Design review of the part built by this model. Coordinates are the model's own, in mm. Give positions to 0.01 mm unless a question says otherwise; leave off trailing zeros. Order: outer loops, then holes, each group sorted by start corner. A loop starts at its lowest first (then second) coordinate and runs counter-clockwise, first axis right, second up. Notation, with made-up numbers: (7.25, -24.5) -> (14.25, -24.5) arc R10 cw to (14.25, -6.5) -> close; hole circle Ø6 at (49, 41). An arc over 180 degrees is marked (long way). One line per item, written item: value. Start each with the question number.
1) Wall thickness on line 1 along X through (y, z) = (18, 0.45); line 2 along Y through (x, z) = (-154, 0.65); line 3 along X through (y, z) = (10, 1.9): over which ranges is each line inside the solid? List them lowest first. Write a range as from..to.
2) Consider section C-C (z = 2.4). State how many separate pieces and enclosed holes the cut face has, plus the area to 3 significant figures.
3) Consider section B-B (x = -20). State the section outline as (y, z) points.
4) Consider section A-A (y = 17.5). State the section outline as (x, z) points, plus the area to 3 significant figures.
Autodesk Fusion 360 part; units mm, degrees
sketch "plate-2026-03-03T15_18_35.082Z" plane through (0, 0, 0) normal (0, 0, 1) x (1, 0, 0)
  line L0 (-7.0864, -44.9336) -> (-7.0864, -31.9336)
  line L1 (6.9136, -44.9336) -> (6.9136, -31.9336)
  line L2 (-6.5864, -45.4336) -> (6.4136, -45.4336)
  line L3 (-6.5864, -31.4336) -> (6.4136, -31.4336)
  arc A0 (-7.0864, -44.9336) -> (-6.5864, -45.4336) centre (-6.5864, -44.9336) ccw
  arc A1 (-6.5864, -31.4336) -> (-7.0864, -31.9336) centre (-6.5864, -31.9336) ccw
  arc A2 (6.4136, -45.4336) -> (6.9136, -44.9336) centre (6.4136, -44.9336) ccw
  arc A3 (6.9136, -31.9336) -> (6.4136, -31.4336) centre (6.4136, -31.9336) ccw
  line L4 (-7.0864, -25.8836) -> (-7.0864, -12.8836)
  line L5 (6.9136, -25.8836) -> (6.9136, -12.8836)
  line L6 (-6.5864, -26.3836) -> (6.4136, -26.3836)
  line L7 (-6.5864, -12.3836) -> (6.4136, -12.3836)
  arc A4 (-7.0864, -25.8836) -> (-6.5864, -26.3836) centre (-6.5864, -25.8836) ccw
  arc A5 (-6.5864, -12.3836) -> (-7.0864, -12.8836) centre (-6.5864, -12.8836) ccw
  arc A6 (6.4136, -26.3836) -> (6.9136, -25.8836) centre (6.4136, -25.8836) ccw
  arc A7 (6.9136, -12.8836) -> (6.4136, -12.3836) centre (6.4136, -12.8836) ccw
  line L8 (-7.0864, -6.8336) -> (-7.0864, 6.1664)
  line L9 (6.9136, -6.8336) -> (6.9136, 6.1664)
  line L10 (-6.5864, -7.3336) -> (6.4136, -7.3336)
  line L11 (-6.5864, 6.6664) -> (6.4136, 6.6664)
  arc A8 (-7.0864, -6.8336) -> (-6.5864, -7.3336) centre (-6.5864, -6.8336) ccw
  arc A9 (-6.5864, 6.6664) -> (-7.0864, 6.1664) centre (-6.5864, 6.1664) ccw
  arc A10 (6.4136, -7.3336) -> (6.9136, -6.8336) centre (6.4136, -6.8336) ccw
  arc A11 (6.9136, 6.1664) -> (6.4136, 6.6664) centre (6.4136, 6.1664) ccw
  line L12 (-7.0864, 12.2164) -> (-7.0864, 25.2164)
  line L13 (6.9136, 12.2164) -> (6.9136, 25.2164)
  line L14 (-6.5864, 11.7164) -> (6.4136, 11.7164)
  line L15 (-6.5864, 25.7164) -> (6.4136, 25.7164)
  arc A12 (-7.0864, 12.2164) -> (-6.5864, 11.7164) centre (-6.5864, 12.2164) ccw
  arc A13 (-6.5864, 25.7164) -> (-7.0864, 25.2164) centre (-6.5864, 25.2164) ccw
  arc A14 (6.4136, 11.7164) -> (6.9136, 12.2164) centre (6.4136, 12.2164) ccw
  arc A15 (6.9136, 25.2164) -> (6.4136, 25.7164) centre (6.4136, 25.2164) ccw
  line L16 (-7.0864, 31.2664) -> (-7.0864, 44.2664)
  line L17 (6.9136, 31.2664) -> (6.9136, 44.2664)
  line L18 (-6.5864, 30.7664) -> (6.4136, 30.7664)
  line L19 (-6.5864, 44.7664) -> (6.4136, 44.7664)
  arc A16 (-7.0864, 31.2664) -> (-6.5864, 30.7664) centre (-6.5864, 31.2664) ccw
  arc A17 (-6.5864, 44.7664) -> (-7.0864, 44.2664) centre (-6.5864, 44.2664) ccw
  arc A18 (6.4136, 30.7664) -> (6.9136, 31.2664) centre (6.4136, 31.2664) ccw
  arc A19 (6.9136, 44.2664) -> (6.4136, 44.7664) centre (6.4136, 44.2664) ccw
  line L20 (9.4386, -47.9586) -> (9.4386, 47.2914)
  line L21 (-9.6114, -47.9586) -> (-9.6114, 47.2914)
  line L22 (9.4386, -47.9586) -> (-9.6114, -47.9586)
  line L23 (9.4386, 47.2914) -> (-9.6114, 47.2914)
sketch "Sketch2" plane through (0, 0, 0) normal (0, 0, 1) x (1, 0, 0)
  line L0 (19.4386, 72.7414) -> (-193.7614, 72.7414)
  line L1 (-193.7614, 72.7414) -> (-193.7614, -62.4586)
  line L2 (-193.7614, -62.4586) -> (19.4386, -62.4586)
  line L3 (19.4386, -62.4586) -> (19.4386, 72.7414)
  line L4 (9.4386, -47.9586) -> (9.4386, 47.2914)
  line L5 (9.4386, -47.9586) -> (-9.6114, -47.9586)
  circle A0 centre (14.4386, 67.7414) radius 1.45
  circle A1 centre (-188.7614, 67.7414) radius 1.45
  circle A2 centre (-188.7614, -57.4586) radius 1.45
  circle A3 centre (14.4386, -57.4586) radius 1.45
  line L6 (-179.2614, 49.9614) -> (-16.0614, 49.9614)
  line L7 (-16.0614, 49.9614) -> (-16.0614, -47.9586)
  line L8 (-16.0614, -47.9586) -> (-179.2614, -47.9586)
  line L9 (-179.2614, -47.9586) -> (-179.2614, 49.9614)
  dimension "d1" = 213.2
  dimension "d2" = 135.2
  dimension "d3" = 10
  dimension "d5" = 2.9
  dimension "d6" = 2.9
  dimension "d7" = 2.9
  dimension "d8" = 2.9
  dimension "d9" = 5
  dimension "d10" = 5
  dimension "d11" = 5
  dimension "d12" = 5
  dimension "d13" = 5
  dimension "d14" = 5
  dimension "d15" = 5
  dimension "d16" = 5
  dimension "d17" = 163.2
  dimension "d18" = 97.92
  dimension "d20" = 14.5
  dimension "d22" = 14.5
  dimension "d23" = 14.5
extrude "Extrude1" add sketch "Sketch2" along normal blind 3
extrude "Extrude2" cut sketch "plate-2026-03-03T15_18_35.082Z" along normal blind 15 contours L0 L1 L2 L3 A0 A1 A2 A3 | L4 L5 L6 L7 A4 A5 A6 A7 | L8 L9 L10 L11 A8 A9 A10 A11 | L12 L13 L14 L15 A12 A13 A14 A15 | L16 L17 L18 L19 A16 A17 A18 A19
equation "d1 = 193.2 mm + 20 mm"
equation "d2 = 115.2 mm + 20 mm"
Checked values:
1. line 1: x = -193.76..-179.26, -16.06..-7.09, 6.91..19.44
1. line 2: y = -62.46..-47.96, 49.96..72.74
1. line 3: x = -193.76..-179.26, -16.06..19.44
2. separate pieces: 1
2. enclosed holes: 10
2. area: 11,800 mm^2
3. outline: (-62.46, 0) -> (-47.96, 0) -> (-47.96, 3) -> (-62.46, 3) -> close; (49.96, 0) -> (72.74, 0) -> (72.74, 3) -> (49.96, 3) -> close
4. outline: (-193.76, 0) -> (-179.26, 0) -> (-179.26, 3) -> (-193.76, 3) -> close; (-16.06, 0) -> (-7.09, 0) -> (-7.09, 3) -> (-16.06, 3) -> close; (6.91, 0) -> (19.44, 0) -> (19.44, 3) -> (6.91, 3) -> close
4. area: 108 mm^2
